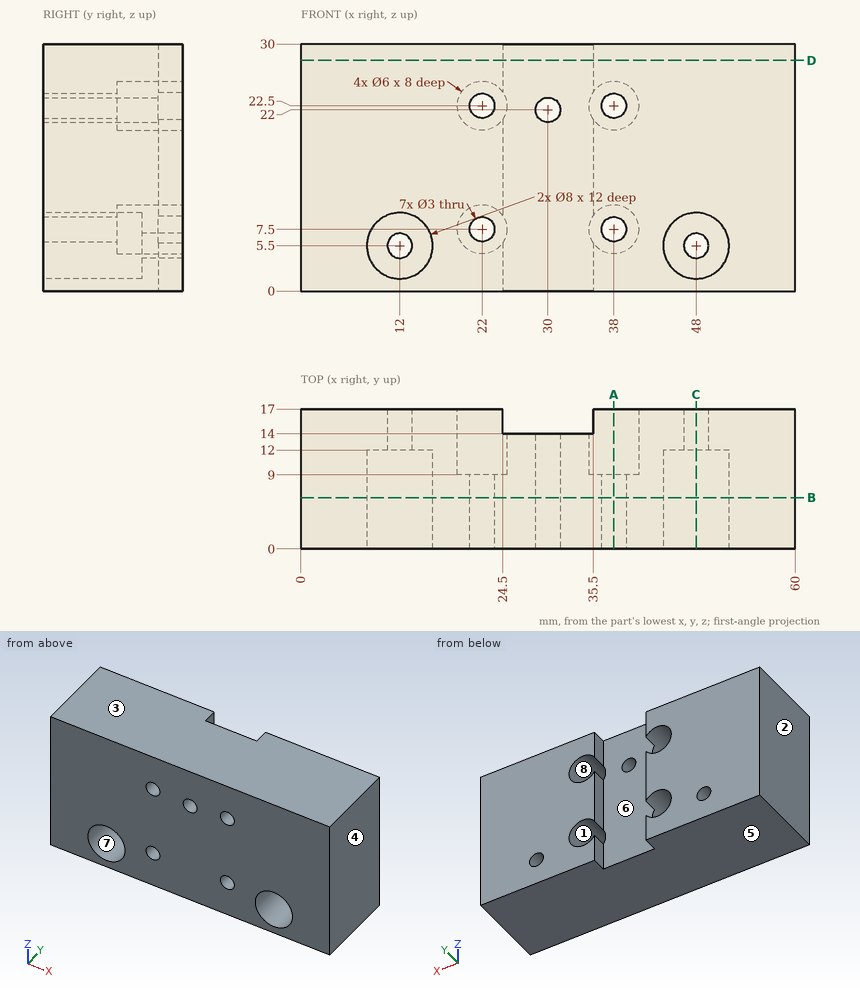
Design review of the part shown in the three views and the two pictorial views. Dimensions are in mm from the part's minimum x, y and z. A direction names the side the tool comes from. Coordinates: 2 decimals unless noted, no trailing zeros. Loops run counter-clockwise (first coordinate to the right, second up) from the corner with the lowest first, then second, coordinate; pieces in that order, holes last. Notation, with made-up numbers: (5, 19.25) - (18, 19.25) arc R12 ccw to (18, 40.25) - close; hole circle Ø8 at (16.25, -37.75). An arc over 180 degrees is marked (long way). Use a Markdown table: item, result. Add a question column.
Item 1: We need section C-C (x = 48). Give the boundary of the cut face in (y, z).
Item 2: Mouldability with a two-part tool opening along Z and no side actions: class the marked faces 1, 2 and 3 as pulls with the +Z half, pulls with the -Z half, needs draft (parallel to the pull), parting line crosses it, or undercut.
Item 3: For line 1 (Z direction, x = 38, y = 7.25); line 2 (X direction, y = 16.5, z = 14); line 3 (X direction, y = 4, z = 22.5), list the stretches that pass through material, from the lowest coordinate up.
Item 4: Tool access review of the marked faces 4, 5, 6, 7 and 8: name each direction out of +Z, -Z, +X, -X, +Y, -Y from which nothing blocks a thin tool from reaching the whole face with its end or side.
Item 5: We need section A-A (x = 38). Give the boundary of the cut face in (y, z).
Item 6: We need section D-D (z = 28). Give the boundary of the cut face in (x, y), and give its area (3 significant figures).
Item 7: Insertion check: pin 1 Ø1.8 at (x, z) = (48, 5.5) entering from +Y; pin 2 Ø1.8 at (x, z) = (39, 7.5) entering from +Y. Each pin has a flat end and moves straight along its axis. Give the tip position at first contact, or say it passes through.
Item 8: We need section B-B (y = 6.25). Give the boundary of the cut face in (x, z), and give its area (3 significant figures).
Results list:
| question | item | result |
|---|---|---|
| 1 | outline | (0, 0) - (17, 0) - (17, 4) - (12, 4) - (12, 1.5) - (0, 1.5) - close; (0, 9.5) - (12, 9.5) - (12, 7) - (17, 7) - (17, 30) - (0, 30) - close |
| 2 | face 1 | undercut |
| 2 | face 2 | needs draft |
| 2 | face 3 | pulls with the +Z half |
| 3 | line 1 | z = 0 to 6, 9 to 21, 24 to 30 |
| 3 | line 2 | x = 0 to 24.5, 35.5 to 60 |
| 3 | line 3 | x = 0 to 20.5, 23.5 to 28.59, 31.41 to 36.5, 39.5 to 60 |
| 4 | face 4 | +Z, -Z, +X, +Y, -Y |
| 4 | face 5 | -Z, +X, -X, +Y, -Y |
| 4 | face 6 | +Z, -Z, +Y |
| 4 | face 7 | -Y |
| 4 | face 8 | +Y |
| 5 | outline | (0, 0) - (17, 0) - (17, 4.5) - (9, 4.5) - (9, 6) - (0, 6) - close; (0, 9) - (9, 9) - (9, 10.5) - (17, 10.5) - (17, 19.5) - (9, 19.5) - (9, 21) - (0, 21) - close; (0, 24) - (9, 24) - (9, 25.5) - (17, 25.5) - (17, 30) - (0, 30) - close |
| 6 | outline | (0, 0) - (60, 0) - (60, 17) - (35.5, 17) - (35.5, 14) - (24.5, 14) - (24.5, 17) - (0, 17) - close |
| 6 | area | 987 mm^2 |
| 7 | pin 1 | passes through |
| 7 | pin 2 | stops at y = 9 |
| 8 | outline | (0, 0) - (60, 0) - (60, 30) - (0, 30) - close; hole circle Ø8 at (12, 5.5); hole circle Ø3 at (22, 7.5); hole circle Ø3 at (22, 22.5); hole circle Ø3 at (30, 22); hole circle Ø3 at (38, 7.5); hole circle Ø3 at (38, 22.5); hole circle Ø8 at (48, 5.5) |
| 8 | area | 1,660 mm^2 |
